Model file for the job. Use its own axes, mm. A direction names the side the tool comes from. Coordinates: 2 decimals unless noted, no trailing zeros. Order: outer loops, then holes, each group sorted by start corner. A loop starts at its lowest first (then second) coordinate and runs counter-clockwise, first axis right, second up.
from build123d import *

# Parameters (mm, degrees)
BOSS_EXTRUDE1_DEPTH      = 6
BOSS_EXTRUDE2_DEPTH      = 28
SKETCH5_W                = 15.5
SKETCH5_H                = 90
CUT_EXTRUDE2_DEPTH       = 273.596771808
CHAMFER2_SIZE            = 3
SKETCH8_W                = 46
SKETCH8_H                = 73
CUT_EXTRUDE4_DEPTH       = 23
BOSS_EXTRUDE5_DEPTH      = 73
BOSS_EXTRUDE5_DEPTH_BACK = 3
BOSS_EXTRUDE5_START      = 114
BOSS_EXTRUDE6_DEPTH      = 18.95
SKETCH11_W               = 31
SKETCH11_H               = 38.46
CUT_EXTRUDE5_DEPTH       = 19.03
CUT_EXTRUDE7_START       = 18.95
CUT_EXTRUDE7_DEPTH       = 20
CUT_EXTRUDE8_REACH       = 274.597
CUT_EXTRUDE9_REACH       = 274.597
SKETCH13_W               = 17.55
SKETCH13_H               = 4
CUT_EXTRUDE10_REACH      = 274.597
SKETCH14_W               = 3
SKETCH14_H               = 3
SKETCH15_W               = 6
SKETCH15_H               = 8
SKETCH15_W_2             = 5.75
SKETCH15_H_2             = 10
CUT_EXTRUDE11_DEPTH      = 2


with BuildPart() as part:
    # Sketch1 → Boss-Extrude1 (new body)
    with BuildSketch(Plane(origin=(0, 0, 0), x_dir=(1, 0, 0), z_dir=(0, 1, 0))):
        Polygon((105, -35), (65, 0), (0, 0), (0, -250), (65, -250), (65, -35), align=None)
        Polygon((0, -250), (0, 0), (-65, 0), (-105, -35), (-65, -35), (-65, -250), align=None)
    extrude(amount=BOSS_EXTRUDE1_DEPTH)

    # Sketch2 → Boss-Extrude2 (add)
    with BuildSketch(Plane(origin=(0, 6, 0), x_dir=(1, 0, 0), z_dir=(0, 1, 0))):
        Polygon((-105, -35), (-97.407038705, -35), (-63.121324419, -5), (63.121324419, -5), (97.407038705, -35), (105, -35), (65, 0), (-65, 0), align=None)
    extrude(amount=BOSS_EXTRUDE2_DEPTH)

    # Sketch5 → Cut-Extrude2 (cut, through all)
    with BuildSketch(Plane(origin=(0, 6, 0), x_dir=(1, 0, 0), z_dir=(0, 1, 0))):
        with Locations((-57.25, -80)):
            Rectangle(SKETCH5_W, SKETCH5_H)
        with Locations((57.25, -80)):
            Rectangle(SKETCH5_W, SKETCH5_H)
    extrude(amount=-CUT_EXTRUDE2_DEPTH, mode=Mode.SUBTRACT)

    # Chamfer2
    chamfer2_edges = [part.edges().sort_by_distance(p)[0] for p in [
        (-65, 3, 125),
        (-49.5, 3, 35),
        (-49.5, 3, 125),
        (65, 3, 125),
        (49.5, 3, 125),
        (49.5, 3, 35),
    ]]
    chamfer(chamfer2_edges, length=CHAMFER2_SIZE)

    # Sketch8 → Cut-Extrude4 (cut)
    with BuildSketch(Plane(origin=(0, 6, 0), x_dir=(1, 0, 0), z_dir=(0, 1, 0))):
        with Locations((0, -150.5)):
            Rectangle(SKETCH8_W, SKETCH8_H)
    extrude(amount=-CUT_EXTRUDE4_DEPTH, mode=Mode.SUBTRACT)

    # Sketch9 → Boss-Extrude5 (add, two sides: drawn at the far end of the back side and taken through both)
    with BuildSketch(Plane.XY.offset(BOSS_EXTRUDE5_START - BOSS_EXTRUDE5_DEPTH_BACK)):
        with BuildLine():
            Line((-27, 12), (-23, 12))
            ThreePointArc((-23, 12), (0, -11), (23, 12))
            Line((23, 12), (27, 12))
            ThreePointArc((27, 12), (0, -15), (-27, 12))
        make_face()
    extrude(amount=BOSS_EXTRUDE5_DEPTH + BOSS_EXTRUDE5_DEPTH_BACK)

    # Sketch10 → Boss-Extrude6 (add)
    with BuildSketch(Plane(origin=(0, 6, 0), x_dir=(1, 0, 0), z_dir=(0, 1, 0))):
        Polygon((-19.35, -250), (-19.35, -207.69), (19.35, -207.69), (19.35, -250), (15.5, -250), (15.5, -211.54), (-15.5, -211.54), (-15.5, -250), align=None)
    extrude(amount=BOSS_EXTRUDE6_DEPTH)

    # Sketch11 → Cut-Extrude5 (cut)
    with BuildSketch(Plane(origin=(0, 6, 0), x_dir=(1, 0, 0), z_dir=(0, 1, 0))):
        with Locations((0, -230.77)):
            Rectangle(SKETCH11_W, SKETCH11_H)
    extrude(amount=-CUT_EXTRUDE5_DEPTH, mode=Mode.SUBTRACT)

    # Sketch10<3> → Cut-Extrude7 (cut)
    with BuildSketch(Plane(origin=(0, 6, 0), x_dir=(1, 0, 0), z_dir=(0, 1, 0)).offset(CUT_EXTRUDE7_START)):
        Polygon((-19.35, -250), (-19.35, -207.69), (19.35, -207.69), (19.35, -250), (15.5, -250), (15.5, -211.54), (-15.5, -211.54), (-15.5, -250), align=None)
    extrude(amount=-CUT_EXTRUDE7_DEPTH, mode=Mode.SUBTRACT)

    # Sketch12 → Cut-Extrude8 (cut, up to next)
    with BuildSketch(Plane(origin=(0, 6, 0), x_dir=(1, 0, 0), z_dir=(0, 1, 0)), mode=Mode.PRIVATE) as cut_extrude8_sk1:
        with BuildLine():
            Line((-11.5, -114), (11.5, -114))
            ThreePointArc((11.5, -114), (0, -107.028878229), (-11.5, -114))
        make_face()
    cut_extrude8_tool1 = extrude(cut_extrude8_sk1.sketch, amount=-CUT_EXTRUDE8_REACH, mode=Mode.PRIVATE) & part.part
    add(cut_extrude8_tool1.solids().sort_by_distance((0, 6, 111.135325))[0], mode=Mode.SUBTRACT)

    # Sketch13 → Cut-Extrude9 (cut, up to next)
    with BuildSketch(Plane(origin=(0, 6, 0), x_dir=(1, 0, 0), z_dir=(0, 1, 0)), mode=Mode.PRIVATE) as cut_extrude9_sk1:
        with Locations((0, -189)):
            Rectangle(SKETCH13_W, SKETCH13_H)
    cut_extrude9_tool1 = extrude(cut_extrude9_sk1.sketch, amount=-CUT_EXTRUDE9_REACH, mode=Mode.PRIVATE) & part.part
    add(cut_extrude9_tool1.solids().sort_by_distance((0, 6, 189))[0], mode=Mode.SUBTRACT)

    # Sketch14 → Cut-Extrude10 (cut, up to next)
    with BuildSketch(Plane(origin=(0, 6, 0), x_dir=(1, 0, 0), z_dir=(0, 1, 0)), mode=Mode.PRIVATE) as cut_extrude10_sk1:
        with Locations((-31.5, -126.5)):
            Rectangle(SKETCH14_W, SKETCH14_H)
    cut_extrude10_tool1 = extrude(cut_extrude10_sk1.sketch, amount=-CUT_EXTRUDE10_REACH, mode=Mode.PRIVATE) & part.part
    # Sketch14 → Cut-Extrude10 (cut, up to next)
    with BuildSketch(Plane(origin=(0, 6, 0), x_dir=(1, 0, 0), z_dir=(0, 1, 0)), mode=Mode.PRIVATE) as cut_extrude10_sk2:
        with Locations((-31.5, -177.5)):
            Rectangle(SKETCH14_W, SKETCH14_H)
    cut_extrude10_tool2 = extrude(cut_extrude10_sk2.sketch, amount=-CUT_EXTRUDE10_REACH, mode=Mode.PRIVATE) & part.part
    # Sketch14 → Cut-Extrude10 (cut, up to next)
    with BuildSketch(Plane(origin=(0, 6, 0), x_dir=(1, 0, 0), z_dir=(0, 1, 0)), mode=Mode.PRIVATE) as cut_extrude10_sk3:
        with Locations((31.5, -126.5)):
            Rectangle(SKETCH14_W, SKETCH14_H)
    cut_extrude10_tool3 = extrude(cut_extrude10_sk3.sketch, amount=-CUT_EXTRUDE10_REACH, mode=Mode.PRIVATE) & part.part
    # Sketch14 → Cut-Extrude10 (cut, up to next)
    with BuildSketch(Plane(origin=(0, 6, 0), x_dir=(1, 0, 0), z_dir=(0, 1, 0)), mode=Mode.PRIVATE) as cut_extrude10_sk4:
        with Locations((31.5, -177.5)):
            Rectangle(SKETCH14_W, SKETCH14_H)
    cut_extrude10_tool4 = extrude(cut_extrude10_sk4.sketch, amount=-CUT_EXTRUDE10_REACH, mode=Mode.PRIVATE) & part.part
    add(cut_extrude10_tool1.solids().sort_by_distance((-31.5, 6, 126.5))[0], mode=Mode.SUBTRACT)
    add(cut_extrude10_tool2.solids().sort_by_distance((-31.5, 6, 177.5))[0], mode=Mode.SUBTRACT)
    add(cut_extrude10_tool3.solids().sort_by_distance((31.5, 6, 126.5))[0], mode=Mode.SUBTRACT)
    add(cut_extrude10_tool4.solids().sort_by_distance((31.5, 6, 177.5))[0], mode=Mode.SUBTRACT)

    # Sketch15 → Cut-Extrude11 (cut)
    with BuildSketch(Plane(origin=(0, 6, 0), x_dir=(1, 0, 0), z_dir=(0, 1, 0))):
        with Locations((-46.5, -104.24941096)):
            Rectangle(SKETCH15_W, SKETCH15_H)
        with Locations((-62.125, -182)):
            Rectangle(SKETCH15_W_2, SKETCH15_H_2)
        with Locations((62.125, -182)):
            Rectangle(SKETCH15_W_2, SKETCH15_H_2)
        with Locations((46.5, -104.24941096)):
            Rectangle(SKETCH15_W, SKETCH15_H)
    extrude(amount=-CUT_EXTRUDE11_DEPTH, mode=Mode.SUBTRACT)


solid = part.part
Q1. Cut at A-A, the plane z = 235. List the corners of the cut face in (x, y).
Established:
outline: (-65, 0) - (-15.5, 0) - (-15.5, 4.95) - (-19.35, 4.95) - (-19.35, 6) - (-65, 6) - close; (15.5, 0) - (65, 0) - (65, 6) - (19.35, 6) - (19.35, 4.95) - (15.5, 4.95) - close
Q2. Mould opens along Z. For faces 6 (the face through (-47, 4, 104)), 7 (the face through (65, 3, 190)), 8 (the face through (-41, 3, 250)) say: pulls with the +Z half, pulls with the -Z half, needs draft (parallel to the pull), parting line crosses it, or undercut.
Established:
face 6: undercut
face 7: needs draft
face 8: pulls with the +Z half
Q3. Which spindle directions (+Z, -Z, +X, -X, +Y, -Y) get a long thin tool onto all of the face, cutting with end or side? Do faces 1 (the face through (0, -12, 187)), 2 (the face through (-80.504, 19.804, 20.21)), 3 (the face through (-65, 3, 188)), 4 (the face through (57, 3, 125)), 5 (the face through (0, 3, 191)). Say none if no direction does.
Established:
face 1: +Z, +X, -X, -Y
face 2: +Z, +Y
face 3: +Z, -X, +Y, -Y
face 4: +X, +Y, -Y
face 5: +Y, -Y
Q4. Probe line 1 (Z direction, x = 57, y = 2); line 2 (Y direction, x = 61.5, z = 193.5); line 3 (X direction, y = 20.5, z = 19.5). List the from-to ranges inside material, lowest first.
Established:
line 1: z = 0 to 35, 125 to 250
line 2: y = 0 to 6
line 3: x = -87.29 to -79.69, 79.69 to 87.29
Q5. Drop flat-ended pins along their axis: P1, Ø1.5, axis at y = 4, z = 127, coming from the -X side; P2, Ø3, axis at y = 3.5, z = 217, coming from the -X side; P3, Ø1.5, axis at y = 3, z = 177.5, coming from the +X side; P4, Ø2, axis at y = -1.5, z = 82.5, coming from the -X side. Give the stop position or say it passes through.
Established:
P1: stops at x = -64.75
P2: stops at x = -65
P3: stops at x = 65
P4: passes through
Q6. Cut at B-B, the plane x = 0. List the corners of the cut face in (y, z), plus the area to 3 significant figures.
Established:
outline: (-15, 111) - (-11, 111) - (-11, 187) - (-15, 187) - close; (0, 0) - (34, 0) - (34, 5) - (6, 5) - (6, 107.03) - (0, 107.03) - close; (0, 191) - (6, 191) - (6, 207.69) - (4.95, 207.69) - (4.95, 211.54) - (0, 211.54) - close
area: 1,210 mm2
Q7. Cut at C-C, the plane y = 15. List the corners of the cut face in (x, z), plus the area to 3 significant figures.
Established:
outline: (-105, 35) - (-65, 0) - (65, 0) - (105, 35) - (97.41, 35) - (63.12, 5) - (-63.12, 5) - (-97.41, 35) - close
area: 1,130 mm2
Q8. Cut at D-D, the plane x = 46.5. List the corners of the cut face in (y, z), plus the area to 3 significant figures.
Established:
outline: (0, 0) - (34, 0) - (34, 5) - (6, 5) - (6, 100.25) - (4, 100.25) - (4, 108.25) - (6, 108.25) - (6, 250) - (0, 250) - close
area: 1,620 mm2
